Autodesk Inventor part; units mm, degrees
ref_plane "YZ Plane" through (0, 0, 0) normal (1, 0, 0) x (0, 1, 0)
ref_plane "XZ Plane" through (0, 0, 0) normal (0, 1, 0) x (-1, 0, 0)
ref_plane "XY Plane" through (0, 0, 0) normal (0, 0, 1) x (1, 0, 0)
sketch "Skizze1" plane through (0, 0, 0) normal (1, 0, 0) x (0, 1, 0)
  line L0 (0, 0) -> (0, -5.5)
  line L1 (2, -7.5) -> (6, -7.5)
  line L2 (7.3, -7.0199) -> (12, -3)
  line L3 (12, -3) -> (6, -3)
  line L4 (6, -3) -> (6, 0)
  line L5 (6, 0) -> (1.5, 0)
  line L6 (1.5, 0) -> (0, 0)
  arc A0 (0, -5.5) -> (2, -7.5) centre (2, -5.5) ccw
  arc A1 (6, -7.5) -> (7.3, -7.0199) centre (6, -5.5) ccw
  dimension "d3" = 3
  dimension "d4" = 6
  dimension "d8" = 2
  dimension "d9" = 6
  dimension "d10" = 7.5
extrude "Extrusion1" add sketch "Skizze1" along normal mid plane 3
sketch "Skizze2" plane through (-1.5, 0, 0) normal (0, 0, 1) x (1, 0, 0)
  circle A0 centre (1.5, 3) radius 1.5
  line L0 (0, 0) -> (3, 0)
  point P0 (1.5, 0)
  point P1 (1.5, 0)
  point P2 (1.5, 0)
  dimension "d13" = 3
  dimension "d14" = 3
extrude "Extrusion2" add sketch "Skizze2" along normal blind 7.5
thread "Gewinde1"
properties part number "1 part 8"
Can you work these out from the model? Positions are in its coordinate system, mm. A direction names the side the tool comes from. Coordinates: 2 decimals unless noted, no trailing zeros. Order: outer loops, then holes, each group sorted by start corner. A loop starts at its lowest first (then second) coordinate and runs counter-clockwise, first axis right, second up. Notation, with made-up numbers: (-37.75, 47.5) -> (-5.75, 47.5) arc R25 ccw to (-5.75, 83.5) -> close; hole circle Ø10 at (83.25, -0.5). An arc over 180 degrees is marked (long way). Use one line per item in the form item = value.
Q1. Which directions (+Z, -Z, +X, -X, +Y, -Y) give clear straight access to the entire face, cutting with the end or side of a thin tool? Please do faces 1 (the face through (-0.021, 9.617, -5.038)), 2 (the face through (0, 6, -2)), 3 (the face through (-0.195, 1.513, 3.698)), 4 (the face through (0, 4, -7.5)), 5 (the face through (0, 1, 0)).
From the geometry:
face_1 = -Z, +X, -X, +Y
face_2 = +Z, +X, -X, +Y
face_3 = +Z
face_4 = -Z, +X, -X, +Y, -Y
face_5 = +Z, -Y
Q2. Imagine slicing it at D-D, the plane x = -0.7. List the corners of the cut face in (y, z) for me.
From the geometry:
outline = (0, -5.5) arc R2 ccw to (2, -7.5) -> (6, -7.5) arc R2 ccw to (7.3, -7.02) -> (12, -3) -> (6, -3) -> (6, 0) -> (4.33, 0) -> (4.33, 7.5) -> (1.67, 7.5) -> (1.67, 0) -> (0, 0) -> close
Q3. Imagine slicing it at A-A, the plane x = 0. List the corners of the cut face in (y, z) for me, then the cut area to 3 significant figures.
From the geometry:
outline = (0, -5.5) arc R2 ccw to (2, -7.5) -> (6, -7.5) arc R2 ccw to (7.3, -7.02) -> (12, -3) -> (6, -3) -> (6, 0) -> (4.5, 0) -> (4.5, 7.5) -> (1.5, 7.5) -> (1.5, 0) -> (0, 0) -> close
area = 81.7 mm²
Q4. Imagine slicing it at C-C, the plane y = 3.5. List the corners of the cut face in (x, z) for me, then the cut area to 3 significant figures.
From the geometry:
outline = (-1.5, -7.5) -> (1.5, -7.5) -> (1.5, 0) -> (1.41, 0) -> (1.41, 7.5) -> (-1.41, 7.5) -> (-1.41, 0) -> (-1.5, 0) -> close
area = 43.7 mm²
Q5. I need wall thicknesses on L1, parallel to Z at x = -1.25, y = 5.25; L2, parallel to Y at x = 0.35, z = -2.5; L3, parallel to Y at x = 1.05, z = 3.5. Which ranges of each line are inside material? Lowest first, please.
From the geometry:
L1 = -7.5 to 0
L2 = 0 to 6
L3 = 1.93 to 4.07
Q6. Imagine slicing it at B-B, the plane z = 6.25. List the corners of the cut face in (x, y) for me.
From the geometry:
outline = circle Ø3 at (0, 3)
Q7. Will this pin go through, and if not, where does the flat tip stop? P1, Ø1.5, axis at x = 0, z = -2, coming from the +Y side.
From the geometry:
P1 = 6
